Work out the finished part from the listing and answer in its coordinate system (mm). Give positions to 0.01 mm unless a question says otherwise; leave off trailing zeros. Loops run counter-clockwise (first coordinate to the right, second up) from the corner with the lowest first, then second, coordinate; pieces in that order, holes last.
```python
from build123d import *

# Parameters (mm, degrees)
EXTRUDE_1_DEPTH     = 5
SKETCH_2_R          = 3
CUT_EXTRUDE_2_DEPTH = 27.115129714
SKETCH_3_R          = 1.5
CUT_EXTRUDE_3_DEPTH = 100


with BuildPart() as part:
    # 草圖1 → 伸長1 (new body)
    with BuildSketch(Plane.XY):
        with BuildLine():
            Line((-3.880570001, 20.9701425), (-8.880570001, 0.9701425))
            ThreePointArc((-8.880570001, 0.9701425), (-9, 0), (-8.880570001, -0.9701425))
            Line((-8.880570001, -0.9701425), (-3.880570001, -20.9701425))
            ThreePointArc((-3.880570001, -20.9701425), (0, -24), (3.880570001, -20.9701425))
            Line((3.880570001, -20.9701425), (8.880570001, -0.9701425))
            ThreePointArc((8.880570001, -0.9701425), (9, 0), (8.880570001, 0.9701425))
            Line((8.880570001, 0.9701425), (3.880570001, 20.9701425))
            ThreePointArc((3.880570001, 20.9701425), (0, 24), (-3.880570001, 20.9701425))
        make_face()
    extrude(amount=EXTRUDE_1_DEPTH)

    # 草圖2 → 伸長2 (cut, through all)
    with BuildSketch(Plane.XY.offset(5)):
        Circle(SKETCH_2_R)
    extrude(amount=-CUT_EXTRUDE_2_DEPTH, mode=Mode.SUBTRACT)

    # 草圖3 → 伸長3 (cut)
    with BuildSketch(Plane.XY.offset(5)):
        with Locations((0, 15)):
            Circle(SKETCH_3_R)
        with Locations((0, -15)):
            Circle(SKETCH_3_R)
    extrude(amount=-CUT_EXTRUDE_3_DEPTH, mode=Mode.SUBTRACT)


solid = part.part
```
Q1. Section B-B on y = 0 is taken. Give the vertices of the cut face in (x, z), plus the area to 3 significant figures.
Q2. Consider line 1 along Y through (x, z) = (0, 3.55); line 2 along X through (y, z) = (12, 3.9); line 3 along X through (y, z) = (-15.5, 1.9). Determine where each line is inside the solid, lowest interval first.
Q3. Section D-D on y = -15 is taken. Give the vertices of the cut face in (x, z), plus the area to 3 significant figures.
Q4. Section C-C on z = 4.45 is taken. Give the vertices of the cut face in (x, y), plus the area to 3 significant figures.
Q5. Section A-A on x = 0 is taken. Give the vertices of the cut face in (y, z).
Q6. Determine the mould class of faces 1 (the face through (-6.346, 11.11, 2.465)), 2 (the face through (-4, 0, 0)), 3 (the face through (9, 0, 2)), 4 (the face through (-0.325, -16.464, 2.535)) for opening direction Y: +Y half, -Y half, draft (parallel to the pull), parting line (faces both ways), or undercut.
Check result:
1. outline: (-9, 0) - (-3, 0) - (-3, 5) - (-9, 5) - close; (3, 0) - (9, 0) - (9, 5) - (3, 5) - close
1. area: 60.0 mm2
2. line 1: y = -24 to -16.5, -13.5 to -3, 3 to 13.5, 16.5 to 24
2. line 2: x = -6.12 to 6.12
2. line 3: x = -5.25 to -1.41, 1.41 to 5.25
3. outline: (-5.37, 0) - (-1.5, 0) - (-1.5, 5) - (-5.37, 5) - close; (1.5, 0) - (5.37, 0) - (5.37, 5) - (1.5, 5) - close
3. area: 38.7 mm2
4. outline: (-8.88, -0.97) - (-3.88, -20.97) arc R4 ccw to (3.88, -20.97) - (8.88, -0.97) arc R4 ccw to (8.88, 0.97) - (3.88, 20.97) arc R4 ccw to (-3.88, 20.97) - (-8.88, 0.97) arc R4 ccw to start; hole circle Ø6 at (0, 0); hole circle Ø3 at (0, -15); hole circle Ø3 at (0, 15)
4. area: 538 mm2
5. outline: (-24, 0) - (-16.5, 0) - (-16.5, 5) - (-24, 5) - close; (-13.5, 0) - (-3, 0) - (-3, 5) - (-13.5, 5) - close; (3, 0) - (13.5, 0) - (13.5, 5) - (3, 5) - close; (16.5, 0) - (24, 0) - (24, 5) - (16.5, 5) - close
6. face 1: +Y half
6. face 2: draft
6. face 3: parting line
6. face 4: undercut
